Source: CAD feature listing. Evaluate the final solid. Frame: model axes, mm. A direction names the side the tool comes from. Coordinates: 2 decimals unless noted, no trailing zeros. Loops run counter-clockwise (first coordinate to the right, second up) from the corner with the lowest first, then second, coordinate; pieces in that order, holes last.
from build123d import *

# Parameters (mm, degrees)
F0_R     = 24
F0_R_2   = 3
F1_DEPTH = 3
F2_DEPTH = 30
F0_W     = 62
F0_H     = 62
F3_DEPTH = 25
F4_R     = 2
F5_R     = 2
F6_SIZE  = 2


with BuildPart() as f1:
    # F0 (on Top) → F1 (new body)
    with BuildSketch(Plane.XY):
        Circle(F0_R)
        Circle(F0_R_2, mode=Mode.SUBTRACT)
        Circle(F0_R_2)
    extrude(amount=F1_DEPTH)

    # F0 (on Top) → F2 (join)
    with BuildSketch(Plane.XY):
        Circle(F0_R_2)
    extrude(amount=F2_DEPTH)

    # F0 (on Top) → F3 (join)
    with BuildSketch(Plane.XY):
        Rectangle(F0_W, F0_H)
        Circle(F0_R, mode=Mode.SUBTRACT)
        Circle(F0_R)
        Circle(F0_R_2, mode=Mode.SUBTRACT)
        Circle(F0_R_2)
    extrude(amount=-F3_DEPTH)

    # F4
    f4_edges = [f1.edges().sort_by_distance(p)[0] for p in [
        (31, -31, -12.5),
        (31, 31, -12.5),
        (-31, -31, -12.5),
        (-31, 31, -12.5),
    ]]
    fillet(f4_edges, radius=F4_R)

    # F5
    f5_edges = [f1.edges().sort_by_distance(p)[0] for p in [
        (-24, 0, 3),
    ]]
    fillet(f5_edges, radius=F5_R)

    # F6
    f6_edges = [f1.edges().sort_by_distance(p)[0] for p in [
        (-3, 0, 30),
    ]]
    chamfer(f6_edges, length=F6_SIZE)


solid = f1.part
Q1. Line query: line 1 along Z through (x, y) = (17.5, -10); line 2 along Z through (x, y) = (-26, 20); line 3 along Y through (x, z) = (18, 2). Output: solid intervals per line, ascending.
Q2. Section D-D, the plane y = -27. Return the cut outline in (x, z).
Q3. Section C-C, the plane z = 23. Return the cut outline in (x, y), plus the area to 3 significant figures.
Q4. Section A-A, the plane y = 0. Return the cut outline in (x, z).
Q5. Access query for faces 1 (the cylindrical face through (-3, 0, 15)), 2 (the cylindrical face through (30.4, -30.43, -12.68)). Directions: +Z, -Z, +X, -X, +Y, -Y. A direction counts if a zero-diameter tool reaches every point of the face in a straight line with its end or side. Return the directions, or none.
Q6. Contact query for a flat-ended pin moving along its axis: pin 1 Ø10 at (x, y) = (19.5, 19.5) entering from +Z. Output: stop coordinate, or through.
Derived:
1. line 1: z = -25 to 3
1. line 2: z = -25 to 0
1. line 3: y = -15.47 to 15.47
2. outline: (-31, -25) - (31, -25) - (31, 0) - (-31, 0) - close
3. outline: circle Ø6 at (0, 0)
3. area: 28.3 mm2
4. outline: (-31, -25) - (31, -25) - (31, 0) - (24, 0) - (24, 1) arc R2 ccw to (22, 3) - (3, 3) - (3, 28) - (1, 30) - (-1, 30) - (-3, 28) - (-3, 3) - (-22, 3) arc R2 ccw to (-24, 1) - (-24, 0) - (-31, 0) - close
5. face 1: +Z
5. face 2: +Z, -Z, +X, -Y
6. pin 1: stops at z = 2.91
